Verification items for the finished model (mm, model axes). A direction names the side the tool comes from. Give positions to 0.01 mm unless a question says otherwise; leave off trailing zeros. Order: outer loops, then holes, each group sorted by start corner. A loop starts at its lowest first (then second) coordinate and runs counter-clockwise, first axis right, second up. Notation, with made-up numbers: (-12.75, 32.25) - (15.25, 32.25) arc R26 cw to (15.25, 54.25) - close; hole circle Ø10 at (7.5, 34.25). An arc over 180 degrees is marked (long way). Answer as a JSON object with one key per item and string values.
```python
from build123d import *

# Parameters (mm, degrees)
SKETCH1_R           = 10.2
BOSS_EXTRUDE1_DEPTH = 20.1
CUT_EXTRUDE3_DEPTH  = 21.1
SKETCH9_R           = 12.5
BOSS_EXTRUDE3_DEPTH = 8
SKETCH10_R          = 4
BOSS_EXTRUDE4_DEPTH = 5
CUT_EXTRUDE5_DEPTH  = 15
SKETCH12_R          = 6.5
BOSS_EXTRUDE5_DEPTH = 6


with BuildPart() as part:
    # Sketch1 → Boss-Extrude1 (new body)
    with BuildSketch(Plane(origin=(0, 0, 0), x_dir=(1, 0, 0), z_dir=(0, 1, 0))):
        Circle(SKETCH1_R)
    extrude(amount=BOSS_EXTRUDE1_DEPTH)

    # Sketch6 → Cut-Extrude3 (cut, through all)
    with BuildSketch(Plane(origin=(0, 20.1, 0), x_dir=(1, 0, 0), z_dir=(0, 1, 0))):
        Polygon((-3.6, 6.86312611), (3.6, 6.86312611), (5.03591293, 8.870151124), (5.03591293, 10.936036024), (-4.887797844, 10.936036024), (-5.03591293, 8.870151124), align=None)
    extrude(amount=-CUT_EXTRUDE3_DEPTH, mode=Mode.SUBTRACT)

    # Sketch9 → Boss-Extrude3 (add)
    with BuildSketch(Plane(origin=(0, 20.1, 0), x_dir=(1, 0, 0), z_dir=(0, 1, 0))):
        Circle(SKETCH9_R)
    extrude(amount=BOSS_EXTRUDE3_DEPTH)

    # Sketch10 → Boss-Extrude4 (add)
    with BuildSketch(Plane(origin=(0, 28.1, 0), x_dir=(1, 0, 0), z_dir=(0, 1, 0))):
        Circle(SKETCH10_R)
    extrude(amount=BOSS_EXTRUDE4_DEPTH)

    # Sketch11 → Cut-Extrude5 (cut)
    with BuildSketch(Plane(origin=(0, 33.1, 0), x_dir=(1, 0, 0), z_dir=(0, 1, 0))):
        with BuildLine():
            Line((-1.29614814, 1.1), (1.29614814, 1.1))
            ThreePointArc((1.29614814, 1.1), (0, -1.7), (-1.29614814, 1.1))
        make_face()
    extrude(amount=-CUT_EXTRUDE5_DEPTH, mode=Mode.SUBTRACT)

    # Sketch12 → Boss-Extrude5 (add)
    with BuildSketch(Plane.XZ):
        Circle(SKETCH12_R)
    extrude(amount=BOSS_EXTRUDE5_DEPTH)


solid = part.part
```
(1) Release check for a two-part mould opening along Z. For faces 1 (the flat face through (0, 18.1, 0)), 2 (the flat face through (0, 0, 7)), 3 (the flat face through (-4.328, 10.191, -7.881)) record: pulls with the +Z half, pulls with the -Z half, needs draft (parallel to the pull), parting line crosses it, or undercut.
Computed values:
{"face 1": "undercut", "face 2": "needs draft", "face 3": "pulls with the -Z half"}
(2) Access from +Z, -Z, +X, -X, +Y, -Y to the whole of each face (thin tool, end or side, straight path). Record for faces 4 (the flat face through (0, 10, -6.863)), 5 (the cylindrical face through (-5.158, -2.958, -3.955)), 6 (the cylindrical face through (-0.867, 30.565, 3.905)), 7 (the flat face through (0, -6, 0)).
Computed values:
{"face 4": "-Z, -Y", "face 5": "-Y", "face 6": "+Y", "face 7": "+Z, -Z, +X, -X, -Y"}
(3) Section check D-D (y = 24). Record the cut outline in (x, z).
Computed values:
{"outline": "circle Ø25 at (0, 0); hole (-1.3, -1.1) - (1.3, -1.1) arc R1.7 ccw (long way) to start"}
(4) Section check A-A (x = 0). Record the cut outline in (y, z).
Computed values:
{"outline": "(-6, -6.5) - (0, -6.5) - (0, -6.86) - (20.1, -6.86) - (20.1, -12.5) - (28.1, -12.5) - (28.1, -4) - (33.1, -4) - (33.1, -1.1) - (18.1, -1.1) - (18.1, 1.7) - (33.1, 1.7) - (33.1, 4) - (28.1, 4) - (28.1, 12.5) - (20.1, 12.5) - (20.1, 10.2) - (0, 10.2) - (0, 6.5) - (-6, 6.5) - close"}
(5) Section check C-C (y = -1.5). Record the cut outline in (x, z), then the cut area to 3 significant figures.
Computed values:
{"outline": "circle Ø13 at (0, 0)", "area": "133 mm²"}
(6) Section check B-B (z = 0). Record the cut outline in (x, y), then the cut area to 3 significant figures.
Computed values:
{"outline": "(-12.5, 20.1) - (-10.2, 20.1) - (-10.2, 0) - (-6.5, 0) - (-6.5, -6) - (6.5, -6) - (6.5, 0) - (10.2, 0) - (10.2, 20.1) - (12.5, 20.1) - (12.5, 28.1) - (4, 28.1) - (4, 33.1) - (1.7, 33.1) - (1.7, 18.1) - (-1.7, 18.1) - (-1.7, 33.1) - (-4, 33.1) - (-4, 28.1) - (-12.5, 28.1) - close", "area": "677 mm²"}
(7) Gauge pin test, flat ends, axial feed: pin 1 Ø6 at (x, z) = (-8, 7) entering from -Y; pin 2 Ø3 at (x, y) = (-3, 16) entering from -Z; pin 3 Ø5 at (x, y) = (2, 9) entering from +Z. Record the tip position at first contact, or that the pin passes through.
Computed values:
{"pin 1": "stops at y = 0", "pin 2": "stops at z = -8.12", "pin 3": "stops at z = 10.2"}
(8) Material ranges on line 1 along X through (y, z) = (23, 0); line 2 along Y through (x, z) = (-6, -7); line 3 along Y through (x, z) = (4.25, -9.25), recorded low to high. Write a range as [from, to].
Computed values:
{"line 1": "x = [-12.5, -1.7], [1.7, 12.5]", "line 2": "y = [0, 28.1]", "line 3": "y = [20.1, 28.1]"}
